For this review, take the finished solid that the model builds, in its own axes (mm). A direction names the side the tool comes from. Round coordinates to 2 decimals unless told otherwise and drop trailing zeros. Write each loop counter-clockwise with the first axis right and the second up, starting at its lowest first coordinate (ties: lowest second). Pieces come first, ordered by that corner, then holes. Notation, with made-up numbers: (85, 83.5) -> (144, 83.5) arc R35 cw to (144, 118.5) -> close; hole circle Ø10 at (-33.75, 14.25). An arc over 180 degrees is marked (long way). Answer in a Markdown table with one row per item. Add a question column.
```python
from build123d import *

# Parameters (mm, degrees)
BOSS_EXTRUDE1_DEPTH = 19.5
SKETCH3_W           = 18.5
SKETCH3_H           = 22
BOSS_EXTRUDE2_DEPTH = 25
SKETCH5_W           = 50
SKETCH5_H           = 15
SKETCH5_W_2         = 15
SKETCH5_H_2         = 5
CUT_EXTRUDE1_DEPTH  = 40.5
BOSS_EXTRUDE4_DEPTH = 3.5
BOSS_EXTRUDE5_DEPTH = 3.5
BOSS_EXTRUDE6_DEPTH = 3.5
FILLET3_R           = 3
SKETCH12_R          = 1.7
CUT_EXTRUDE4_DEPTH  = 5
SKETCH13_R          = 1.7
CUT_EXTRUDE5_DEPTH  = 45
SKETCH14_R          = 1.7
CUT_EXTRUDE6_DEPTH  = 45
SKETCH15_R          = 1.7
CUT_EXTRUDE7_DEPTH  = 4
FILLET4_R           = 1


with BuildPart() as part:
    # Sketch1 → Boss-Extrude1 (new body)
    with BuildSketch(Plane.XY):
        Polygon((-5.699410772, 32.916253451), (16.300589228, 32.916253451), (16.300589228, -23.083746549), (-5.699410772, -23.083746549), (-5.699410772, 10.916253451), (-37.199410772, 10.916253451), (-37.199410772, 32.916253451), align=None)
    extrude(amount=BOSS_EXTRUDE1_DEPTH)

    # Sketch3 → Boss-Extrude2 (add)
    with BuildSketch(Plane.XY.offset(19.5)):
        with Locations((7.050589228, 21.916253451)):
            Rectangle(SKETCH3_W, SKETCH3_H)
    extrude(amount=BOSS_EXTRUDE2_DEPTH)

    # Sketch5 → Cut-Extrude1 (cut)
    with BuildSketch(Plane.XY.offset(44.5)):
        with Locations((-12.199410772, 21.916253451)):
            Rectangle(SKETCH5_W, SKETCH5_H)
        with Locations((5.300589228, -3.083746549)):
            Rectangle(SKETCH5_W_2, SKETCH5_H)
        with Locations((5.300589228, -17.083746549)):
            Rectangle(SKETCH5_W_2, SKETCH5_H_2)
    extrude(amount=-CUT_EXTRUDE1_DEPTH, mode=Mode.SUBTRACT)

    # Sketch7 → Boss-Extrude4 (add)
    with BuildSketch(Plane(origin=(16.300589228, 0, 0), x_dir=(0, 0, -1), z_dir=(1, 0, 0))):
        with BuildLine():
            Line((-34.5, 10.916253451), (-19.5, 10.916253451))
            Line((-19.5, 10.916253451), (-19.5, -4.083746549))
            ThreePointArc((-19.5, -4.083746549), (-23.893398282, 6.522855169), (-34.5, 10.916253451))
        make_face()
    extrude(amount=-BOSS_EXTRUDE4_DEPTH)

    # Sketch8 → Boss-Extrude5 (add)
    with BuildSketch(Plane(origin=(0, 0, 0), x_dir=(-1, 0, 0), z_dir=(0, 0, -1))):
        with BuildLine():
            Line((5.699410772, 10.916253451), (20.699410772, 10.916253451))
            ThreePointArc((20.699410772, 10.916253451), (10.092809055, 6.522855169), (5.699410772, -4.083746549))
            Line((5.699410772, -4.083746549), (5.699410772, 10.916253451))
        make_face()
    extrude(amount=-BOSS_EXTRUDE5_DEPTH)

    # Sketch9 → Boss-Extrude6 (add)
    with BuildSketch(Plane(origin=(0, 32.916253451, 0), x_dir=(1, 0, 0), z_dir=(0, 1, 0))):
        with BuildLine():
            Line((-2.199410772, -34.5), (-2.199410772, -19.5))
            Line((-2.199410772, -19.5), (-17.199410772, -19.5))
            ThreePointArc((-17.199410772, -19.5), (-6.592809055, -23.893398282), (-2.199410772, -34.5))
        make_face()
    extrude(amount=-BOSS_EXTRUDE6_DEPTH)

    # Fillet3
    fillet3_edges = [part.edges().sort_by_distance(p)[0] for p in [
        (-2.199410772, 12.666253451, 19.5),
    ]]
    fillet(fillet3_edges, radius=FILLET3_R)

    # Sketch12 → Cut-Extrude4 (cut)
    with BuildSketch(Plane(origin=(0, 0, 0), x_dir=(-1, 0, 0), z_dir=(0, 0, -1))):
        with Locations((-5.300589228, 21.916253451)):
            Circle(SKETCH12_R)
        with Locations((10.949410772, 21.916253451)):
            Circle(SKETCH12_R)
        with Locations((27.199410772, 21.916253451)):
            Circle(SKETCH12_R)
    extrude(amount=-CUT_EXTRUDE4_DEPTH, mode=Mode.SUBTRACT)

    # Sketch13 → Cut-Extrude5 (cut)
    with BuildSketch(Plane.ZY.offset(5.699410772)):
        with Locations(Location((10.5, -3.083746549, 0), (0, 0, 270))):
            Circle(SKETCH13_R)
    extrude(amount=-CUT_EXTRUDE5_DEPTH, mode=Mode.SUBTRACT)

    # Sketch14 → Cut-Extrude6 (cut)
    with BuildSketch(Plane(origin=(16.300589228, 0, 0), x_dir=(0, 0, -1), z_dir=(1, 0, 0))):
        with Locations(Location((-10.5, 21.916253451, 0), (0, 0, 90))):
            Circle(SKETCH14_R)
        with Locations(Location((-35.5, 21.916253451, 0), (0, 0, 90))):
            Circle(SKETCH14_R)
    extrude(amount=-CUT_EXTRUDE6_DEPTH, mode=Mode.SUBTRACT)

    # Sketch15 → Cut-Extrude7 (cut)
    with BuildSketch(Plane.XZ.offset(23.083746549)):
        with Locations(Location((5.300589228, 9.75, 0), (0, 0, 270))):
            Circle(SKETCH15_R)
    extrude(amount=-CUT_EXTRUDE7_DEPTH, mode=Mode.SUBTRACT)

    # Fillet4
    fillet4_edges = [part.edges().sort_by_distance(p)[0] for p in [
        (-5.699410772, -13.583746549, 0),
        (-10.092809055, 6.522855169, 0),
        (-27.199410772, 32.916253451, 19.5),
        (-6.592809055, 32.916253451, 23.893398282),
        (16.300589228, 32.916253451, 22.25),
        (-37.199410772, 32.916253451, 9.75),
        (16.300589228, -13.583746549, 19.5),
        (16.300589228, 10.916253451, 39.5),
        (-2.199410772, 32.916253451, 39.5),
        (16.300589228, 21.916253451, 44.5),
        (7.050589228, 32.916253451, 44.5),
        (-10.449410772, 32.916253451, 0),
        (16.300589228, 4.916253451, 0),
        (-28.949410772, 10.916253451, 0),
        (-37.199410772, 21.916253451, 0),
        (16.300589228, 6.522855169, 23.893398282),
    ]]
    fillet(fillet4_edges, radius=FILLET4_R)


solid = part.part
```
1. Tool access review of faces 1 (the cylindrical face through (14.575, 20.218, 10.575)), 2 (the flat face through (-7, 29.416, 19)), 3 (the flat face through (-27, 31, 19.5)), 4 (the flat face through (5, -14.584, 12)), 5 (the flat face through (-9, 8, 3.5)): name each direction out of +Z, -Z, +X, -X, +Y, -Y from which nothing blocks a thin tool from reaching the whole face with its end or side.
2. Clearance check with flat-ended pins moving along their axes: pin 1 Ø5.5 at (x, y) = (7, -17) entering from +Z; pin 2 Ø1.5 at (x, y) = (-30, 25) entering from +Z; pin 3 Ø0.8 at (y, z) = (31.5, 39.5) entering from -X; pin 4 Ø2.5 at (y, z) = (-3.08, 10.5) entering from -X. State where each tip first meets the part, or that it passes through.
3. We need section B-B (x = 1.5). Write out the cut boundary in (y, z).
4. We need section A-A (z = 35.5). Write out the cut boundary in (x, y).
5. We need section C-C (z = 9.75). Count the separate pieces of the cut face and the enclosed holes in it, plus the area to 3 significant figures.
6. The part is to be moulded in two halves that separate along Y. For faces 6 (the flat face through (5, 4.416, 12)), 7 (the flat face through (-2.199, 13, 33)), 8 (the flat face through (5, -23.084, 12)), say which applies: pulls with the +Y half, pulls with the -Y half, needs draft (parallel to the pull), parting line crosses it, or undercut.
7. For L1, parallel to Y at x = -1, z = 12; L2, parallel to Y at x = 2.5, z = 30; L3, parallel to X at y = -3, z = 13.5, list the stretches that pass through material, from the lowest coordinate up. Write a range as [from, to].
Response:
| question | item | result |
|---|---|---|
| 1 | face 1 | +X, -X |
| 1 | face 2 | +Z, -X |
| 1 | face 3 | +Z, -X, +Y, -Y |
| 1 | face 4 | +Z |
| 1 | face 5 | +Z, -X, -Y |
| 2 | pin 1 | z = 19.5 |
| 2 | pin 2 | z = 4 |
| 2 | pin 3 | x = -2.2 |
| 2 | pin 4 | through |
| 3 | outline | (-23.08, 0) -> (31.92, 0) arc R1 ccw to (32.92, 1) -> (32.92, 43.5) arc R1 ccw to (31.92, 44.5) -> (29.42, 44.5) -> (29.42, 4) -> (14.42, 4) -> (14.42, 44.5) -> (10.92, 44.5) -> (10.92, 19.5) -> (4.42, 19.5) -> (4.42, 4) -> (-10.58, 4) -> (-10.58, 19.5) -> (-14.58, 19.5) -> (-14.58, 4) -> (-19.58, 4) -> (-19.58, 19.5) -> (-23.08, 19.5) -> close |
| 4 | outline | (-2.2, 10.92) -> (15.3, 10.92) arc R1 ccw to (16.3, 11.92) -> (16.3, 20.22) -> (12.8, 20.22) -> (12.8, 14.42) -> (-2.2, 14.42) -> close; (-2.2, 29.42) -> (12.8, 29.42) -> (12.8, 23.62) -> (16.3, 23.62) -> (16.3, 31.92) arc R1 ccw to (15.3, 32.92) -> (-1.2, 32.92) arc R1 ccw to (-2.2, 31.92) -> close |
| 5 | separate pieces | 3 |
| 5 | enclosed holes | 0 |
| 5 | area | 831 mm2 |
| 6 | face 6 | undercut |
| 6 | face 7 | needs draft |
| 6 | face 8 | pulls with the -Y half |
| 7 | L1 | [-23.08, -19.58], [-14.58, -10.58], [4.42, 14.42], [29.42, 32.92] |
| 7 | L2 | [10.92, 14.42], [29.42, 32.92] |
| 7 | L3 | [-5.7, -2.2], [12.8, 16.3] |
